Solid Edge part; units mm, degrees
sketch "Sketch1" plane through (0, 0, 0) normal (0, -1, 0) x (1, 0, 0)
  line L0 (0, 0) -> (0, -2.75)
  line L1 (0, -2.75) -> (3, -2.75)
  line L2 (3, -2.75) -> (3, -1.5)
  line L3 (3, -1.5) -> (27.6935, -1.5)
  line L4 (27.6935, -1.5) -> (28, -1.1935)
  line L5 (28, -1.1935) -> (28, 0)
  line L6 (28, 0) -> (0, 0)
revolve "RevolvedProtrusion1" add sketch "Sketch1" angle 360 about axis through (28, 0, 0) along (-1, 0, 0)
cosmetic_thread "Thread1"
sketch "Sketch2" plane through (0, 0, 0) normal (-1, 0, 0) x (0, -1, 0)
  line L0 (-0.7217, 1.25) -> (-1.4434, 0)
  line L1 (-1.4434, 0) -> (-0.7217, -1.25)
  line L2 (-0.7217, -1.25) -> (0.7217, -1.25)
  line L3 (0.7217, -1.25) -> (1.4434, 0)
  line L4 (1.4434, 0) -> (0.7217, 1.25)
  line L5 (0.7217, 1.25) -> (-0.7217, 1.25)
extrude "ExtrudedCutout_1" cut sketch "Sketch2" against normal blind 1.3
properties part number "CQ-M3X25L"
Part model, mm, in its own coordinate system. A direction names the side the tool comes from. Give positions to 0.01 mm unless a question says otherwise; leave off trailing zeros. Loops run counter-clockwise (first coordinate to the right, second up) from the corner with the lowest first, then second, coordinate; pieces in that order, holes last. Notation, with made-up numbers: M -19.75,29.25 L -5.75,29.25 A10 ccw -5.75,35.25 Z; hole C 23.25,45 d4. An arc over 180 degrees is marked long. Put each result on its own line as item: value. Start each with the question number.
1) 3-axis set-ups, long thin cutter, end or side, ignore diameter. For faces 1 (the flat face through (0, -1.3, -0.6)), 2 (the cylindrical face through (15.52, 0.07, 1.5)), 3 (the flat face through (0.64, 1.08, 0.63)): which of +Z, -Z, +X, -X, +Y, -Y reach the whole face in a straight line?
2) Pull direction Y, two halves, no side cores. Call faces 4 (the flat face through (3, 1.2, -1.2)), 5 (the cylindrical face through (1.521, -2.685, 0.596)), 6 (the flat face through (1.3, 0, 0)): +Y half, -Y half, draft (parallel to the pull), parting line (faces both ways), or undercut.
3) Saw through at C-C (z = -2.05). List the corners of the cut face in (x, y), then the cut area to 3 significant figures.
4) Saw through at B-B (x = 3.5). List the corners of the cut face in (y, z), then the cut area to 3 significant figures.
5) Saw through at A-A (y = 0). List the corners of the cut face in (x, z).
6) Probe probe 1 along X at (y, z) = (-0.3, 0.6); probe 2 along X at (y, z) = (-1.35, 0.85); probe 3 along Z at (x, y) = (9.25, 0). List the from-to ranges inside material, lowest first.
7) Flat gauge pins, fed straight in: pin 1 (1 mm diameter, centred on x = 5.5, z = -1, fed in from +Y); pin 2 (2 mm diameter, centred on x = 19, y = -2, fed in from -Z); pin 3 (0.8 mm diameter, centred on y = 0, z = -0.5, fed in from -X). Where does each tip first touch, or does it go through?
Numbers:
1. face 1: +Z, -Z, -X, +Y, -Y
1. face 2: +X
1. face 3: -X
2. face 4: draft
2. face 5: parting line
2. face 6: undercut
3. outline: M 0,-1.83 L 3,-1.83 L 3,1.83 L 0,1.83 Z
3. area: 11.0 mm^2
4. outline: C 0,0 d3
4. area: 7.07 mm^2
5. outline: M 0,-2.75 L 3,-2.75 L 3,-1.5 L 27.69,-1.5 L 28,-1.19 L 28,1.19 L 27.69,1.5 L 3,1.5 L 3,2.75 L 0,2.75 L 0,1.25 L 1.3,1.25 L 1.3,-1.25 L 0,-1.25 Z
6. probe 1: 1.3 to 28
6. probe 2: 0 to 3
6. probe 3: -1.5 to 1.5
7. pin 1: y = 1.41
7. pin 2: z = -1.12
7. pin 3: x = 1.3
